Can you work these out from the model? Positions are in its coordinate system, mm. Face numbers are marked on the shaded views. Round coordinates to 2 decimals unless told otherwise and drop trailing zeros. Order: outer loops, then holes, each group sorted by start corner. A loop starts at its lowest first (then second) coordinate and runs counter-clockwise, first axis right, second up.
Q1. If I drill on line 1 (Y direction, x = 12.5, z = 2.75); line 2 (Y direction, x = 11.25, z = 2.75); line 3 (X direction, y = 7.25, z = 4), over which ranges is the centre line in solid material (lowest first)?
Q2. If we section it at A-A (y = 7.5): Please give me the cut outline in (x, z), plus the area to 3 significant figures.
Q3. We'd pull the mould along Y, two halves only. Please class the marked faces 1, 2, 3 and 4: pulls with the +Y half, pulls with the -Y half, needs draft (parallel to the pull), parting line crosses it, or undercut.
Q4. If we section it at C-C (z = 1.75): Please give me the cut outline in (x, y).
Q5. If we section it at B-B (x = 12.5): Please give me the cut outline in (y, z), plus the area to 3 significant figures.
Q6. Will this pin go through, and if not, where does the flat tip stop? P1, Ø2.5, axis at x = 12.5, y = 7.5, coming from the -Z side.
Autodesk Inventor part; units mm, degrees
ref_plane "YZ Plane" through (0, 0, 0) normal (1, 0, 0) x (0, 1, 0)
ref_plane "XZ Plane" through (0, 0, 0) normal (0, 1, 0) x (-1, 0, 0)
ref_plane "XY Plane" through (0, 0, 0) normal (0, 0, 1) x (1, 0, 0)
sketch "Sketch1" plane through (0, 0, 0) normal (0, 0, 1) x (1, 0, 0)
  line L0 (0, 0) -> (25, 0)
  line L1 (25, 0) -> (25, 15)
  line L2 (25, 15) -> (0, 15)
  line L3 (0, 15) -> (0, 0)
  circle A0 centre (12.5, 7.5) radius 1.6
  point P0 (0, 7.5)
  point P1 (12.5, 15)
  dimension "d1" = 15
  dimension "d2" = 25
  dimension "d4" = 3.2
extrude "Extrusion1" add sketch "Sketch1" along normal blind 6.731
equation "\"d10\" = THICKB"
equation "\"THICKA\" = 3.175"
equation "\"THICKB\" = 6.731"
equation "\"THICKC\" = 12.7"
equation "\"MAGDIA\" = 9.5"
equation "\"BALLDIA\" = 12"
equation "\"THICKPLY\" = 5"
properties part number "Frame_Upper_Plate_Pulley_B"
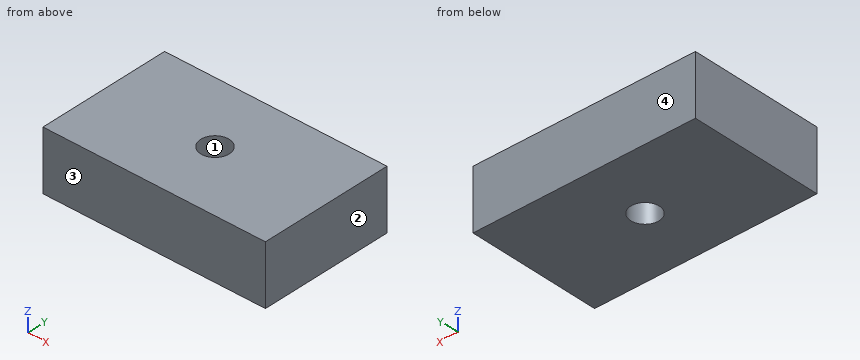
Solution:
1. line 1: y = 0 to 5.9, 9.1 to 15
1. line 2: y = 0 to 6.5, 8.5 to 15
1. line 3: x = 0 to 10.92, 14.08 to 25
2. outline: (0, 0) - (10.9, 0) - (10.9, 6.73) - (0, 6.73) - close; (14.1, 0) - (25, 0) - (25, 6.73) - (14.1, 6.73) - close
2. area: 147 mm2
3. face 1: undercut
3. face 2: needs draft
3. face 3: pulls with the -Y half
3. face 4: pulls with the +Y half
4. outline: (0, 0) - (25, 0) - (25, 15) - (0, 15) - close; hole circle Ø3.2 at (12.5, 7.5)
5. outline: (0, 0) - (5.9, 0) - (5.9, 6.73) - (0, 6.73) - close; (9.1, 0) - (15, 0) - (15, 6.73) - (9.1, 6.73) - close
5. area: 79.4 mm2
6. P1: passes through
